from build123d import *

# Parameters (mm, degrees)
SKETCH1_W           = 3.4
SKETCH1_H           = 8.2
BOSS_EXTRUDE1_DEPTH = 3.175


with BuildPart() as part:
    # Sketch1 → Boss-Extrude1 (new body)
    with BuildSketch(Plane(origin=(0, 0, 0), x_dir=(1, 0, 0), z_dir=(0, 1, 0))):
        with BuildLine():
            ThreePointArc((-22.912878475, -10), (25, 0), (-22.912878475, 10))
            Line((-22.912878475, 10), (-130, 10))
            Line((-130, 10), (-130, -10))
            Line((-130, -10), (-22.912878475, -10))
        make_face()
        with Locations((-123.3, 0)):
            Rectangle(SKETCH1_W, SKETCH1_H, mode=Mode.SUBTRACT)
        with Locations((-98.3, 0)):
            Rectangle(SKETCH1_W, SKETCH1_H, mode=Mode.SUBTRACT)
        with BuildLine():
            Line((-2.7, 6.593604856), (-2.7, 9.5))
            Line((-2.7, 9.5), (2.7, 9.5))
            Line((2.7, 9.5), (2.7, 6.593604856))
            ThreePointArc((2.7, 6.593604856), (0, -7.125), (-2.7, 6.593604856))
        make_face(mode=Mode.SUBTRACT)
    extrude(amount=BOSS_EXTRUDE1_DEPTH)


solid = part.part
Geometry: final body of the model. Coordinates: model frame, mm. A direction names the side the tool comes from. Give positions to 0.01 mm unless a question says otherwise; leave off trailing zeros. Loops run counter-clockwise (first coordinate to the right, second up) from the corner with the lowest first, then second, coordinate; pieces in that order, holes last. Notation, with made-up numbers: (76, 68) -> (97, 68) arc R29 ccw to (97, 103) -> close; hole circle Ø6 at (16.5, 37.5). An arc over 180 degrees is marked (long way). Put each result on its own line as item: value.
1. Pin query (flat end, axial travel): P1, Ø1, axis at x = -91, y = 1.5, coming from the -Z side; P2, Ø1.6, axis at x = -65.5, y = 2, coming from the +Z side; P3, Ø1, axis at y = 2, z = 0.5, coming from the +X side. Return the tip coordinate at first contact, or that it passes through.
Taken from the geometry:
P1: stops at z = -10
P2: stops at z = 10
P3: stops at x = 25
2. Cut plane B-B (z = 0). Return the cut outline in (x, y) (3 decimals), plus the area to 3 significant figures.
Taken from the geometry:
outline: (-130, 0) -> (-125, 0) -> (-125, 3.175) -> (-130, 3.175) -> close; (-121.6, 0) -> (-100, 0) -> (-100, 3.175) -> (-121.6, 3.175) -> close; (-96.6, 0) -> (-7.125, 0) -> (-7.125, 3.175) -> (-96.6, 3.175) -> close; (7.125, 0) -> (25, 0) -> (25, 3.175) -> (7.125, 3.175) -> close
area: 425 mm2
3. Set-up query: faces 5 (the flat face through (-77, 2, 10)), 6 (the flat face through (-36, 3.175, 0)), 7 (the flat face through (-96.6, 2, 0)), 8 (the flat face through (-76, 2, -10)). Return all of +Z, -Z, +X, -X, +Y, -Y with unobstructed straight access to the full face (end or side cutting, diameter ignored); none if empty.
Taken from the geometry:
face 5: +Z, -X, +Y, -Y
face 6: +Z, -Z, +X, -X, +Y
face 7: +Y, -Y
face 8: -Z, -X, +Y, -Y
4. Cut plane C-C (y = 0.7). Return the cut outline in (x, z) (3 decimals).
Taken from the geometry:
outline: (-130, -10) -> (-22.913, -10) arc R25 ccw (long way) to (-22.913, 10) -> (-130, 10) -> close; hole (-125, -4.1) -> (-121.6, -4.1) -> (-121.6, 4.1) -> (-125, 4.1) -> close; hole (-100, -4.1) -> (-96.6, -4.1) -> (-96.6, 4.1) -> (-100, 4.1) -> close; hole (-2.7, -9.5) -> (2.7, -9.5) -> (2.7, -6.594) arc R7.125 ccw (long way) to (-2.7, -6.594) -> close
5. Pull-direction query (X, two-part tool) for faces 1 (the cylindrical face through (24.98, 1.57, 0.96)), 2 (the flat face through (-100, 2, 0)), 3 (the flat face through (-130, 2, 0)), 4 (the flat face through (2.7, 2, -8)); classes: released by +X, released by -X, zero draft, split by the parting line, or undercut.
Taken from the geometry:
face 1: split by the parting line
face 2: undercut
face 3: released by -X
face 4: undercut
6. Cut plane A-A (x = 0). Return the cut outline in (y, z) (3 decimals), plus the area to 3 significant figures.
Taken from the geometry:
outline: (0, -25) -> (3.175, -25) -> (3.175, -9.5) -> (0, -9.5) -> close; (0, 7.125) -> (3.175, 7.125) -> (3.175, 25) -> (0, 25) -> close
area: 106 mm2
7. Ray query, line 1 along X through (y, z) = (0.8, 0) (3 decimals); line 2 along Z through (x, y) = (-36, 1.8); line 3 along X through (y, z) = (2.25, -6). Return the intervals inside material, ascending. Write a range as [from, to].
Taken from the geometry:
line 1: x = [-130, -125], [-121.6, -100], [-96.6, -7.125], [7.125, 25]
line 2: z = [-10, 10]
line 3: x = [-130, -3.84], [3.84, 24.27]
8. Cut plane D-D (x = -71.5). Return the cut outline in (y, z) (3 decimals), plus the area to 3 significant figures.
Taken from the geometry:
outline: (0, -10) -> (3.175, -10) -> (3.175, 10) -> (0, 10) -> close
area: 63.5 mm2
